Design review of the part built by this model. Coordinates are the model's own, in mm. Coordinates: 2 decimals unless noted, no trailing zeros. Write each loop counter-clockwise with the first axis right and the second up, starting at its lowest first coordinate (ties: lowest second). Pieces come first, ordered by that corner, then holes.
Q1. Take a section at B-B, the plane z = -43.25. Write out the cut boundary in (x, y), plus the area to 3 significant figures.
Q2. Take a section at A-A, the plane x = -55.75. Write out the cut boundary in (y, z).
Q3. The part is to be moulded in two halves that separate along Z. For faces 1 (the cylindrical face through (-57.342, 1.268, -40.859)), 2 (the flat face through (-51, 1, -52.075)), 3 (the flat face through (-43, 2.5, -42)), say which applies: released by +Z, released by -Z, zero draft, split by the parting line, or undercut.
Q4. For L1, parallel to X at y = 1.35, z = -41.5; L2, parallel to Z at x = -47.25, y = 1.7; L3, parallel to Z at x = -47.5, y = 0.4, list the stretches that pass through material, from the lowest coordinate up.
Q5. For pin 1 Ø3.5 at (x, z) = (-45.75, -42.08) entering from +Y, flat-tipped, find the tip position at first contact; note if it passes through.
Q6. Take a section at C-C, the plane y = 0.8. Write out the cut boundary in (x, z).
Q7. Take a section at D-D, the plane x = -46. Write out the cut boundary in (y, z).
from build123d import *

# Parameters (mm, degrees)
SKETCH1_W           = 20
SKETCH1_H           = 20
BOSS_EXTRUDE1_DEPTH = 2.5
SKETCH2_R           = 0.6858
CUT_EXTRUDE1_DEPTH  = 21
SKETCH3_R           = 2
CUT_EXTRUDE2_DEPTH  = 3.5


with BuildPart() as part:
    # Sketch1 → Boss-Extrude1 (new body)
    with BuildSketch(Plane(origin=(0, 0, 0), x_dir=(1, 0, 0), z_dir=(0, 1, 0))):
        with Locations((-50.754716981, 42.075471698)):
            Rectangle(SKETCH1_W, SKETCH1_H)
    extrude(amount=BOSS_EXTRUDE1_DEPTH)

    # Sketch2 → Cut-Extrude1 (cut, through all)
    with BuildSketch(Plane.XY.offset(-32.075471698)):
        with Locations((-50.754716981, 2.75)):
            Circle(SKETCH2_R)
    extrude(amount=-CUT_EXTRUDE1_DEPTH, mode=Mode.SUBTRACT)

    # Sketch3 → Cut-Extrude2 (cut, through all)
    with BuildSketch(Plane(origin=(0, 2.5, 0), x_dir=(1, 0, 0), z_dir=(0, 1, 0))):
        with Locations((-55.754716981, 42.075471698)):
            Circle(SKETCH3_R)
        with Locations((-45.754716981, 42.075471698)):
            Circle(SKETCH3_R)
    extrude(amount=-CUT_EXTRUDE2_DEPTH, mode=Mode.SUBTRACT)


solid = part.part
Responses:
1. outline: (-60.75, 0) - (-57.37, 0) - (-57.37, 2.5) - (-60.75, 2.5) - close; (-54.14, 0) - (-47.37, 0) - (-47.37, 2.5) - (-50.12, 2.5) arc R0.69 cw to (-51.39, 2.5) - (-54.14, 2.5) - close; (-44.14, 0) - (-40.75, 0) - (-40.75, 2.5) - (-44.14, 2.5) - close
1. area: 33.4 mm2
2. outline: (0, -52.08) - (2.5, -52.08) - (2.5, -44.08) - (0, -44.08) - close; (0, -40.08) - (2.5, -40.08) - (2.5, -32.08) - (0, -32.08) - close
3. face 1: undercut
3. face 2: released by -Z
3. face 3: zero draft
4. L1: x = -60.75 to -57.67, -53.84 to -47.67, -43.84 to -40.75
4. L2: z = -52.08 to -43.4, -40.75 to -32.08
4. L3: z = -52.08 to -43.05, -41.1 to -32.08
5. pin 1: passes through
6. outline: (-60.75, -52.08) - (-40.75, -52.08) - (-40.75, -32.08) - (-60.75, -32.08) - close; hole circle Ø4 at (-55.75, -42.08); hole circle Ø4 at (-45.75, -42.08)
7. outline: (0, -52.08) - (2.5, -52.08) - (2.5, -44.06) - (0, -44.06) - close; (0, -40.09) - (2.5, -40.09) - (2.5, -32.08) - (0, -32.08) - close
